```python
from build123d import *

# Parameters (mm, degrees)
SKETCH1_R           = 1.65
BOSS_EXTRUDE1_DEPTH = 5
SKETCH2_W           = 36
SKETCH2_H           = 36
BOSS_EXTRUDE2_DEPTH = 1.8
CUT_EXTRUDE1_REACH  = 58.399
SKETCH3_W           = 5
SKETCH3_H           = 3.2
FILLET1_R           = 1


with BuildPart() as part:
    # Sketch1 → Boss-Extrude1 (new body)
    with BuildSketch(Plane(origin=(0, 0, 0), x_dir=(1, 0, 0), z_dir=(0, 1, 0))):
        with BuildLine():
            Line((-28, -24), (28, -24))
            Line((28, -24), (28, 17.89570392))
            ThreePointArc((28, 17.89570392), (0, 24.701428863), (-28, 17.89570392))
            Line((-28, 17.89570392), (-28, -24))
        make_face()
        with Locations(Location((-24, 16, 0), (0, 0, 270))):
            Circle(SKETCH1_R, mode=Mode.SUBTRACT)
        with Locations(Location((24, 16, 0), (0, 0, 270))):
            Circle(SKETCH1_R, mode=Mode.SUBTRACT)
        with Locations(Location((-24, -20, 0), (0, 0, 270))):
            Circle(SKETCH1_R, mode=Mode.SUBTRACT)
        with Locations(Location((24, -20, 0), (0, 0, 270))):
            Circle(SKETCH1_R, mode=Mode.SUBTRACT)
        Polygon((20.1, -20.1), (20.1, 21.1), (18.1, 21.1), (18.1, 20.1), (-18.1, 20.1), (-18.1, 21.1), (-20.1, 21.1), (-20.1, -20.1), align=None, mode=Mode.SUBTRACT)
    extrude(amount=BOSS_EXTRUDE1_DEPTH)

    # Sketch2 → Boss-Extrude2 (add)
    with BuildSketch(Plane(origin=(0, 5, 0), x_dir=(1, 0, 0), z_dir=(0, 1, 0))):
        Polygon((-20.1, 21.1), (-20.1, -20.1), (20.1, -20.1), (20.1, 21.1), (18.1, 21.1), (18.1, 20.1), (-18.1, 20.1), (-18.1, 21.1), align=None)
        Rectangle(SKETCH2_W, SKETCH2_H, mode=Mode.SUBTRACT)
    extrude(amount=-BOSS_EXTRUDE2_DEPTH)

    # Sketch3 → Cut-Extrude1 (cut, up to next)
    with BuildSketch(Plane.XY.offset(24), mode=Mode.PRIVATE) as cut_extrude1_sk1:
        with Locations((-17.6, 1.6)):
            Rectangle(SKETCH3_W, SKETCH3_H)
    cut_extrude1_tool1 = extrude(cut_extrude1_sk1.sketch, amount=-CUT_EXTRUDE1_REACH, mode=Mode.PRIVATE) & part.part
    # Sketch3 → Cut-Extrude1 (cut, up to next)
    with BuildSketch(Plane.XY.offset(24), mode=Mode.PRIVATE) as cut_extrude1_sk2:
        with Locations((17.6, 1.6)):
            Rectangle(SKETCH3_W, SKETCH3_H)
    cut_extrude1_tool2 = extrude(cut_extrude1_sk2.sketch, amount=-CUT_EXTRUDE1_REACH, mode=Mode.PRIVATE) & part.part
    add(cut_extrude1_tool1.solids().sort_by_distance((-17.6, 1.6, 24))[0], mode=Mode.SUBTRACT)
    add(cut_extrude1_tool2.solids().sort_by_distance((17.6, 1.6, 24))[0], mode=Mode.SUBTRACT)

    # Fillet1
    fillet1_edges = [part.edges().sort_by_distance(p)[0] for p in [
        (-18, 4.1, 18),
        (18, 4.1, 18),
        (18, 4.1, -18),
        (-18, 4.1, -18),
        (-20.1, 1.6, -21.1),
        (-18.1, 1.6, -21.1),
        (18.1, 1.6, -21.1),
        (20.1, 1.6, -21.1),
    ]]
    fillet(fillet1_edges, radius=FILLET1_R - 0.0001)  # a hair under: the kernel refuses the full size


solid = part.part
```
For this review, take the finished solid that the model builds, in its own axes (mm). A direction names the side the tool comes from. Give positions to 0.01 mm unless a question says otherwise; leave off trailing zeros. Loops run counter-clockwise (first coordinate to the right, second up) from the corner with the lowest first, then second, coordinate; pieces in that order, holes last. Notation, with made-up numbers: M 77.25,-3.75 L 110.25,-3.75 A22 cw 110.25,33.25 Z; hole C -6.5,-5.5 d10. An arc over 180 degrees is marked long. One line per item, written item: value. Start each with the question number.
Q1. Clearance check with flat-ended pins moving along their axes: pin 1 Ø0.9 at (x, y) = (-4, 4.5) entering from -Z; pin 2 Ø2.5 at (x, y) = (2, 2) entering from -Z; pin 3 Ø3 at (x, y) = (9.5, 3.5) entering from -Z. State where each tip first meets the part, or that it passes through.
Q2. Add section A-A (y = 1.05). Count the separate pieces of the cut face and the enclosed holes in it, and give its area (3 significant figures).
Q3. Add section C-C (x = 5). Give the boundary of the cut face in (y, z).
Q4. For L1, parallel to X at y = 3.8, z = -16; L2, parallel to X at y = 1.5, z = 20; L3, parallel to Z at x = 1, y = 1.85, list the stretches that pass through material, from the lowest coordinate up.
Q5. Machinability: for faces 1 (the face through (28, 2, 3)), 2 (the face through (0, 2, 20.1)), 3 (the face through (0, 4, 18)), 4 (the face through (-20.1, 2, 2)), which of the approach directions +Z, -Z, +X, -X, +Y, -Y give a long, thin tool a straight path to every point of the face, cutting with its end or side? Answer none if there is none.
Q6. Add section B-B (z = 4). Give the boundary of the cut face in (x, y).
Q7. Draft analysis for pull direction Z (two halves, no side actions). For faces 5 (the face through (0, 2, 24)), 6 (the face through (-19, 5, -1)), 7 (the face through (25.636, 2.465, 19.785)), 8 (the face through (-18, 4, 0)), state which applies: released by +Z, released by -Z, zero draft, split by the parting line, or undercut.
Q8. Add section D-D (x = 24). Give the boundary of the cut face in (y, z), and give its area (3 significant figures).
Reply:
1. pin 1: z = -24.6
1. pin 2: z = -24.7
1. pin 3: z = -24.17
2. separate pieces: 2
2. enclosed holes: 4
2. area: 911 mm²
3. outline: M 0,-24.5 L 5,-24.5 L 5,-18 L 3.2,-18 L 3.2,-20.1 L 0,-20.1 Z; M 0,20.1 L 3.2,20.1 L 3.2,18 L 5,18 L 5,24 L 0,24 Z
4. L1: -28 to -25.65, -22.35 to -18, 18 to 22.35, 25.65 to 28
4. L2: -28 to -25.65, -22.35 to -20.1, 20.1 to 22.35, 25.65 to 28
4. L3: -24.69 to -20.1, 20.1 to 24
5. face 1: +Z, -Z, +X, +Y, -Y
5. face 2: -Y
5. face 3: +Y, -Y
5. face 4: +Z, -Y
6. outline: M -28,0 L -20.1,0 L -20.1,3.2 L -18,3.2 L -18,5 L -28,5 Z; M 18,3.2 L 20.1,3.2 L 20.1,0 L 28,0 L 28,5 L 18,5 Z
7. face 5: released by +Z
7. face 6: zero draft
7. face 7: undercut
7. face 8: undercut
8. outline: M 0,-19.78 L 5,-19.78 L 5,-17.65 L 0,-17.65 Z; M 0,-14.35 L 5,-14.35 L 5,18.35 L 0,18.35 Z; M 0,21.65 L 5,21.65 L 5,24 L 0,24 Z
8. area: 186 mm²
